Read the model definition and answer for the solid it produces. Units are mm, in the model's axes. Face numbers are marked on the shaded views. A direction names the side the tool comes from. Coordinates: 2 decimals unless noted, no trailing zeros. Loops run counter-clockwise (first coordinate to the right, second up) from the corner with the lowest first, then second, coordinate; pieces in that order, holes last. Notation, with made-up numbers: (-25.75, 85) -> (23.25, 85) arc R25 cw to (23.25, 118) -> close; hole circle Ø1 at (-3.5, 60). An arc over 180 degrees is marked (long way). Answer in a Markdown table with one row per item.
```python
from build123d import *

# Parameters (mm, degrees)
SKETCH1_W           = 19.5
SKETCH1_H           = 30
SKETCH1_R           = 2.25
BOSS_EXTRUDE1_DEPTH = 16.5
SKETCH2_R           = 2.25
BOSS_EXTRUDE2_DEPTH = 22
SKETCH3_R           = 2.25
BOSS_EXTRUDE3_DEPTH = 5


with BuildPart() as part:
    # Sketch1 → Boss-Extrude1 (new body)
    with BuildSketch(Plane(origin=(0, 0, 0), x_dir=(1, 0, 0), z_dir=(0, 1, 0))):
        with Locations((9.75, 15)):
            Rectangle(SKETCH1_W, SKETCH1_H)
        with Locations(Location((9.75, 22.830092663, 0), (0, 0, 270))):
            Circle(SKETCH1_R, mode=Mode.SUBTRACT)
        with Locations(Location((9.75, 7.169907337, 0), (0, 0, 270))):
            Circle(SKETCH1_R, mode=Mode.SUBTRACT)
    extrude(amount=BOSS_EXTRUDE1_DEPTH)

    # Sketch2 → Boss-Extrude2 (add)
    with BuildSketch(Plane(origin=(0, 16.5, 0), x_dir=(1, 0, 0), z_dir=(0, 1, 0))):
        Polygon((0, 30), (-10, 30), (-10, 0), (0, 0), (19.5, 0), (19.5, 30), align=None)
        with Locations(Location((9.75, 22.830092663, 0), (0, 0, 270))):
            Circle(SKETCH2_R, mode=Mode.SUBTRACT)
        with Locations(Location((9.75, 7.169907337, 0), (0, 0, 270))):
            Circle(SKETCH2_R, mode=Mode.SUBTRACT)
    extrude(amount=BOSS_EXTRUDE2_DEPTH)

    # Sketch3 → Boss-Extrude3 (add)
    with BuildSketch(Plane(origin=(0, 38.5, 0), x_dir=(1, 0, 0), z_dir=(0, 1, 0))):
        Polygon((-10, 30), (-50, 30), (-50, 0), (-10, 0), (19.5, 0), (19.5, 30), align=None)
        with Locations(Location((9.75, 22.830092663, 0), (0, 0, 270))):
            Circle(SKETCH3_R, mode=Mode.SUBTRACT)
        with Locations(Location((9.75, 7.169907337, 0), (0, 0, 270))):
            Circle(SKETCH3_R, mode=Mode.SUBTRACT)
    extrude(amount=BOSS_EXTRUDE3_DEPTH)


solid = part.part
```
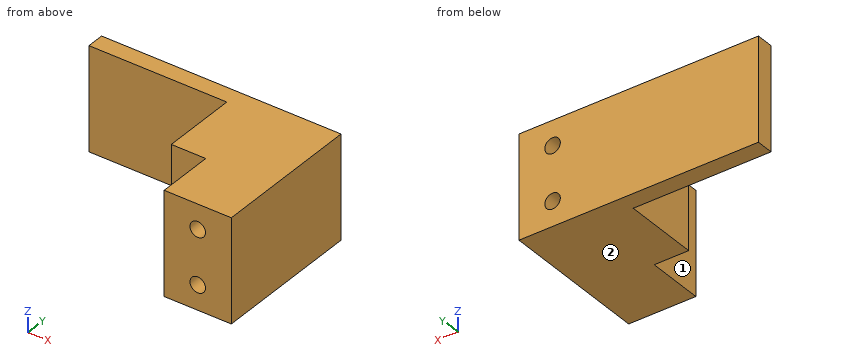
1. A cutting plane is placed at C-C on y = 36. Give the vertices of the cut face in (x, z).
A:
| item | result |
|---|---|
| outline | (-10, -30) -> (19.5, -30) -> (19.5, 0) -> (-10, 0) -> close; hole circle Ø4.5 at (9.75, -22.83); hole circle Ø4.5 at (9.75, -7.17) |
2. Given pin 1 Ø15 at (x, z) = (-34.5, -13) entering from -Y; pin 2 Ø18 at (y, z) = (10, -22.5) entering from -X; pin 3 Ø11 at (x, z) = (-7, -17) entering from -Y, each flat-ended and moving along its own axis, determine where each tip first touches the part or whether it passes through.
A:
| item | result |
|---|---|
| pin 1 | stops at y = 38.5 |
| pin 2 | stops at x = -10 |
| pin 3 | stops at y = 16.5 |
3. A tool of negligible diameter and unlimited length cuts with its end or side. For the marked faces 1 and 2, from which of +Z, -Z, +X, -X, +Y, -Y can it reach the whole face along a straight path? Write none if from no direction.
A:
| item | result |
|---|---|
| face 1 | +Z, -Z, -X, -Y |
| face 2 | -Z, +X, -X, +Y, -Y |
4. A cutting plane is placed at B-B on z = -23.75. Give the vertices of the cut face in (x, y), and give its area (3 significant figures).
A:
| item | result |
|---|---|
| outline | (-50, 38.5) -> (-10, 38.5) -> (-10, 16.5) -> (0, 16.5) -> (0, 0) -> (7.7, 0) -> (7.7, 43.5) -> (-50, 43.5) -> close; (11.8, 0) -> (19.5, 0) -> (19.5, 43.5) -> (11.8, 43.5) -> close |
| area | 1,140 mm2 |
5. Find the intervals of material crossed by probe 1 along Z at (x, y) = (9, 40); probe 2 along X at (y, z) = (29, -25.5); probe 3 along X at (y, z) = (13, -18.5), in increasing order.
A:
| item | result |
|---|---|
| probe 1 | z = -30 to -24.95, -20.71 to -9.29, -5.05 to 0 |
| probe 2 | x = -10 to 19.5 |
| probe 3 | x = 0 to 19.5 |
6. A cutting plane is placed at A-A on x = 9.75. Give the vertices of the cut face in (y, z), and give its area (4 significant figures).
A:
| item | result |
|---|---|
| outline | (0, -30) -> (43.5, -30) -> (43.5, -25.08) -> (0, -25.08) -> close; (0, -20.58) -> (43.5, -20.58) -> (43.5, -9.42) -> (0, -9.42) -> close; (0, -4.92) -> (43.5, -4.92) -> (43.5, 0) -> (0, 0) -> close |
| area | 913.5 mm2 |
7. A cutting plane is placed at D-D on z = -18. Give the vertices of the cut face in (x, y).
A:
| item | result |
|---|---|
| outline | (-50, 38.5) -> (-10, 38.5) -> (-10, 16.5) -> (0, 16.5) -> (0, 0) -> (19.5, 0) -> (19.5, 43.5) -> (-50, 43.5) -> close |
